```python
from build123d import *

# Parameters (mm, degrees)
F0_W     = 86
F0_H     = 3.2
F1_DEPTH = 25
F2_R     = 2.15
F3_DEPTH = 12.5
F4_R     = 2.15
F5_DEPTH = 12.5


with BuildPart() as f1:
    # F0 (on Front) → F1 (new body, symmetric)
    with BuildSketch(Plane.XZ):
        Rectangle(F0_W, F0_H)
    extrude(amount=F1_DEPTH, both=True)

    # F2 (on Top) → F3 (cut, symmetric)
    with BuildSketch(Plane.XY):
        with Locations((-31, -20)):
            Circle(F2_R)
        with Locations((31, -20)):
            Circle(F2_R)
        with Locations((-31, 20)):
            Circle(F2_R)
        with Locations((31, 20)):
            Circle(F2_R)
    extrude(amount=F3_DEPTH, both=True, mode=Mode.SUBTRACT)

    # F4 (on Top) → F5 (cut, symmetric)
    with BuildSketch(Plane.XY):
        with Locations((-21.15, 10)):
            Circle(F4_R)
        with Locations((-21.15, -10)):
            Circle(F4_R)
        with Locations((21.15, 10)):
            Circle(F4_R)
        with Locations((21.15, -10)):
            Circle(F4_R)
    extrude(amount=F5_DEPTH, both=True, mode=Mode.SUBTRACT)


solid = f1.part
```
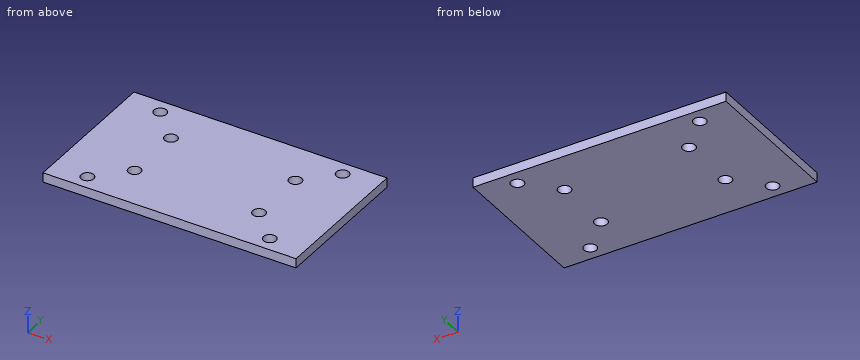
Part model, mm, in its own coordinate system. Round coordinates to 2 decimals unless told otherwise and drop trailing zeros. Loops run counter-clockwise (first coordinate to the right, second up) from the corner with the lowest first, then second, coordinate; pieces in that order, holes last.
1. Slice it at B-B (x = -31). Give the cut face in (y, z), and give its area (3 significant figures).
Solutions:
outline: (-25, -1.6) - (-22.15, -1.6) - (-22.15, 1.6) - (-25, 1.6) - close; (-17.85, -1.6) - (17.85, -1.6) - (17.85, 1.6) - (-17.85, 1.6) - close; (22.15, -1.6) - (25, -1.6) - (25, 1.6) - (22.15, 1.6) - close
area: 132 mm2
2. Slice it at A-A (z = -0.1). Count the separate pieces of the cut face and the enclosed holes in it, and give its area (3 significant figures).
Solutions:
separate pieces: 1
enclosed holes: 8
area: 4,180 mm2
3. Flat gauge pin, fed straight in: pin 1 (5 mm diameter, centred on x = 31, y = -20, fed in from +Z). Where does the tip first touch, or does it go through?
Solutions:
pin 1: stops at z = 1.6
4. Drill centre lines: line 1 along Y through (x, z) = (21, 0.7); line 2 along X through (y, z) = (-20, -0.8); line 3 along Y through (x, z) = (-31, 0.45). Where is each one in solid material? Low to high.
Solutions:
line 1: y = -25 to -12.14, -7.86 to 7.86, 12.14 to 25
line 2: x = -43 to -33.15, -28.85 to 28.85, 33.15 to 43
line 3: y = -25 to -22.15, -17.85 to 17.85, 22.15 to 25
5. Slice it at C-C (y = 10). Give the cut face in (x, z), and give its area (3 significant figures).
Solutions:
outline: (-43, -1.6) - (-23.3, -1.6) - (-23.3, 1.6) - (-43, 1.6) - close; (-19, -1.6) - (19, -1.6) - (19, 1.6) - (-19, 1.6) - close; (23.3, -1.6) - (43, -1.6) - (43, 1.6) - (23.3, 1.6) - close
area: 248 mm2
